```python
from build123d import *

# Parameters (mm, degrees)
F1_DEPTH  = 42.3
F3_W      = 30.3
F3_H      = 6
F4_DEPTH  = 6
F2_W      = 30.3
F2_H      = 6
F5_DEPTH  = 12
F6_SIZE   = 5.99999
F7_R      = 1.5
F8_DEPTH  = 8.501
F9_R      = 1.5
F10_DEPTH = 8.501
F11_R     = 1.5
F11_R_2   = 15.5
F12_DEPTH = 5
F13_SIZE  = 5


# Not quite as in the source:
# - a fillet or chamfer is up to 0.001 mm smaller than in the source, because OpenCascade refuses the exact size
# - a feature names something its author has since deleted; it is built from what else it names


with BuildPart() as f1:
    # F0 (on Right) → F1 (new body)
    with BuildSketch(Plane.YZ):
        Polygon((-9.5, 9.5), (0, 9.5), (0, 14.5), (-14.5, 14.5), (-20.5, 14.5), (-20.5, 8.5), (-62.8, 8.5), (-62.8, 3.5), (-20.5, 3.5), (-20.5, -2.5), (-14.5, -2.5), (-14.5, -14.5), (0, -14.5), (0, -9.5), (-9.5, -9.5), align=None)
    extrude(amount=F1_DEPTH)

    # F3 (on face) → F4 (cut)
    with BuildSketch(Plane.XZ.offset(14.5)):
        with Locations((21.15, -11.5)):
            Rectangle(F3_W, F3_H)
    extrude(amount=-F4_DEPTH, mode=Mode.SUBTRACT)

    # F2 (on face) → F5 (cut)
    with BuildSketch(Plane.XZ.offset(20.5)):
        with Locations((21.15, 11.5)):
            Rectangle(F2_W, F2_H)
    extrude(amount=-F5_DEPTH, mode=Mode.SUBTRACT)

    # F6 (size 6 in the source; OpenCascade refuses exactly that, so slightly less here)
    f6_edges = [f1.edges().sort_by_distance(p)[0] for p in [
        (3, -14.5, -14.5),
        (39.3, -14.5, -14.5),
        (3, -20.5, 14.5),
        (39.3, -20.5, 14.5),
        (21.15, -20.5, -2.5),
    ]]
    chamfer(f6_edges, length=F6_SIZE)

    # F7 (on face) → F8 (cut, through all)
    with BuildSketch(Plane.XZ.offset(8.5)):
        with Locations((10.5, 12)):
            Circle(F7_R)
        with Locations((31.8, 12)):
            Circle(F7_R)
    extrude(amount=-F8_DEPTH, mode=Mode.SUBTRACT)

    # F9 (on face) → F10 (cut, through all)
    with BuildSketch(Plane.XZ.offset(8.5)):
        with Locations((10.5, -12)):
            Circle(F9_R)
        with Locations((31.8, -12)):
            Circle(F9_R)
    extrude(amount=-F10_DEPTH, mode=Mode.SUBTRACT)

    # F11 (on face) → F12 (cut, through all)
    with BuildSketch(Plane.XY.offset(8.5)):
        with Locations((5.65, -57.15)):
            Circle(F11_R)
        with Locations((5.65, -26.15)):
            Circle(F11_R)
        with Locations((36.65, -26.15)):
            Circle(F11_R)
        with Locations((36.65, -57.15)):
            Circle(F11_R)
        with Locations((21.15, -41.65)):
            Circle(F11_R_2)
    extrude(amount=-F12_DEPTH, mode=Mode.SUBTRACT)

    # F13
    f13_edges = [f1.edges().sort_by_distance(p)[0] for p in [
        (42.3, -62.8, 6),
        (0, -62.8, 6),
    ]]
    chamfer(f13_edges, length=F13_SIZE)


solid = f1.part
```
Verification items for the finished model (mm, model axes). A direction names the side the tool comes from. Round coordinates to 2 decimals unless told otherwise and drop trailing zeros. Write each loop counter-clockwise with the first axis right and the second up, starting at its lowest first coordinate (ties: lowest second). Pieces come first, ordered by that corner, then holes.
1. Scan lines: L1, parallel to Z at x = 31.8, y = -5.25; L2, parallel to Z at x = 31, y = -5; L3, parallel to Y at x = 13.5, z = -3. Record each from-to range of solid material in increasing order.
2. Section check C-C on x = 34. State how many separate pieces and enclosed holes the cut face has, plus the area to 3 significant figures.
3. Draft check along Y on faces 1 (the cylindrical face through (38.036, -26.725, 6.035)), 2 (the flat face through (21, -9.5, 0)), 3 (the flat face through (21, -12, -8.5)). Enter one of: +Y half, -Y half, draft (parallel to the pull), parting line (faces both ways), or undercut.
4. Section check B-B on y = -6. Enter the section's corners in (x, z).
5. Section check D-D on y = -53. Enter the section's corners in (x, z), plus the area to 3 significant figures.
6. Gauge pin test, flat ends, axial feed: P1, Ø1.5, axis at x = 14, z = 12, coming from the -Y side; P2, Ø2.5, axis at x = 21, y = -11.5, coming from the -Z side; P3, Ø6, axis at x = 37, y = -19.5, coming from the -Z side. Record the tip position at first contact, or that the pin passes through.
7. Access from +Z, -Z, +X, -X, +Y, -Y to the whole of each face (thin tool, end or side, straight path). Record for faces 4 (the flat face through (11, -28, 3.5)), 5 (the flat face through (21, -5, 9.5)), 6 (the flat face through (21, -24, 8.5)), 7 (the flat face through (21, -8.5, 12)).
8. Section check A-A on z = 12. Enter the section's corners in (x, y).
Answer:
1. L1: z = -14.5 to -13.5, -10.5 to -9.5, 9.5 to 10.5, 13.5 to 14.5
1. L2: z = -14.5 to -13.27, -10.73 to -9.5, 9.5 to 10.73, 13.27 to 14.5
1. L3: y = -14.5 to -9.5
2. separate pieces: 4
2. enclosed holes: 0
2. area: 343 mm2
3. face 1: undercut
3. face 2: +Y half
3. face 3: draft
4. outline: (0, -14.5) - (42.3, -14.5) - (42.3, -9.5) - (0, -9.5) - close; (0, 9.5) - (42.3, 9.5) - (42.3, 14.5) - (0, 14.5) - close; hole circle Ø3 at (10.5, -12); hole circle Ø3 at (10.5, 12); hole circle Ø3 at (31.8, -12); hole circle Ø3 at (31.8, 12)
5. outline: (0, 3.5) - (10.59, 3.5) - (10.59, 8.5) - (0, 8.5) - close; (31.71, 3.5) - (42.3, 3.5) - (42.3, 8.5) - (31.71, 8.5) - close
5. area: 106 mm2
6. P1: stops at y = -8.5
6. P2: stops at z = -8.5
6. P3: stops at z = -0.5
7. face 4: -Z, +X, -X, -Y
7. face 5: +X, -X, +Y
7. face 6: +Z, -Y
7. face 7: +Z, -Z, -Y
8. outline: (0, -17) - (6, -17) - (6, -8.5) - (9, -8.5) - (9, 0) - (0, 0) - close; (12, -8.5) - (30.3, -8.5) - (30.3, 0) - (12, 0) - close; (33.3, -8.5) - (36.3, -8.5) - (36.3, -17) - (42.3, -17) - (42.3, 0) - (33.3, 0) - close
